from build123d import *

# Parameters (mm, degrees)
SKETCH1_R                   = 2.540797377
SKETCH1_W                   = 50.8
SKETCH1_H                   = 22.225
BOSS_EXTRUDE1_DEPTH         = 6.35
F_1_4_0_25_DIAMETER_HOLE1_D = 6.35


with BuildPart() as part:
    # Sketch1 → Boss-Extrude1 (new body)
    with BuildSketch(Plane.XY):
        with Locations((12.7, 0)):
            Circle(SKETCH1_R)
        Rectangle(SKETCH1_W, SKETCH1_H)
        with Locations((12.7, 0)):
            Circle(SKETCH1_R, mode=Mode.SUBTRACT)
    extrude(amount=BOSS_EXTRUDE1_DEPTH)

    # 1/4 (0.25) Diameter Hole1 (through all)
    with Locations(Plane(origin=(0, 0, 0), x_dir=(-1, 0, 0), z_dir=(0, 0, -1))):
        with Locations((-12.7, 0)):
            Hole(F_1_4_0_25_DIAMETER_HOLE1_D / 2)


solid = part.part
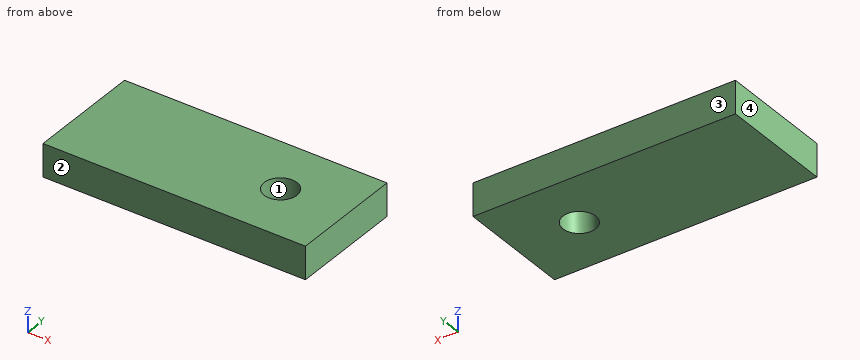
Model file for the job. Use its own axes, mm. Face numbers are marked on the shaded views. Coordinates: 2 decimals unless noted, no trailing zeros. Write each loop counter-clockwise with the first axis right and the second up, starting at its lowest first coordinate (ties: lowest second). Pieces come first, ordered by that corner, then holes. Notation, with made-up numbers: (-5.75, 16) -> (34.25, 16) arc R15 cw to (34.25, 25) -> close; hole circle Ø5 at (20.25, 15). An arc over 180 degrees is marked (long way). One line per item, written item: value. Start each with the question number.
1) Pull direction Y, two halves, no side cores. Call the marked faces 1, 2, 3 and 4: +Y half, -Y half, draft (parallel to the pull), parting line (faces both ways), or undercut.
2) Flat gauge pin, fed straight in: pin 1 Ø5.5 at (x, y) = (12.7, 0) entering from +Z. Where does the tip first touch, or does it go through?
3) Probe probe 1 along Y at (x, z) = (12.7, 5.25) (1 decimal); probe 2 along X at (y, z) = (-0.75, 2.5); probe 3 along X at (y, z) = (2, 3.75). List the from-to ranges inside material, lowest first.
4) Slice it at A-A on y = 0. Write the cut outline in (x, z) (3 decimals), then the cut area to 3 significant figures.
Answers follow:
1. face 1: undercut
1. face 2: -Y half
1. face 3: +Y half
1. face 4: draft
2. pin 1: through
3. probe 1: -11.1 to -3.2, 3.2 to 11.1
3. probe 2: -25.4 to 9.61, 15.79 to 25.4
3. probe 3: -25.4 to 10.23, 15.17 to 25.4
4. outline: (-25.4, 0) -> (9.525, 0) -> (9.525, 6.35) -> (-25.4, 6.35) -> close; (15.875, 0) -> (25.4, 0) -> (25.4, 6.35) -> (15.875, 6.35) -> close
4. area: 282 mm2
